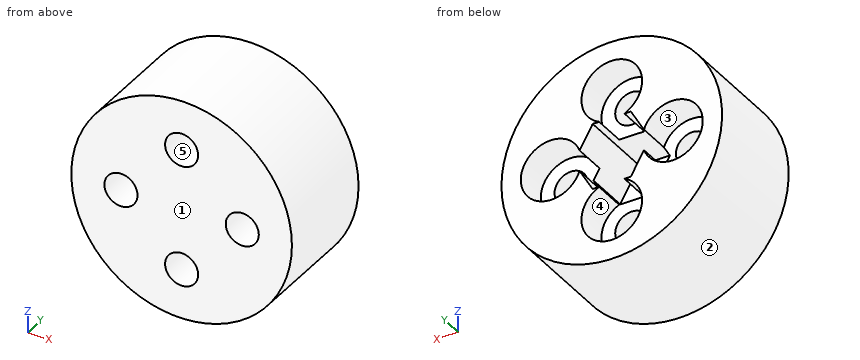
from build123d import *

# Parameters (mm, degrees)
SKETCH1_R           = 10
SKETCH1_R_2         = 1.5
BOSS_EXTRUDE1_DEPTH = 10
SKETCH2_R           = 2.75
CUT_EXTRUDE1_DEPTH  = 3
CUT_EXTRUDE2_DEPTH  = 7


with BuildPart() as part:
    # Sketch1 → Boss-Extrude1 (new body)
    with BuildSketch(Plane(origin=(0, 0, 0), x_dir=(1, 0, 0), z_dir=(0, 1, 0))):
        Circle(SKETCH1_R)
        with Locations((0, 5.5)):
            Circle(SKETCH1_R_2, mode=Mode.SUBTRACT)
        with Locations((5.5, 0)):
            Circle(SKETCH1_R_2, mode=Mode.SUBTRACT)
        with Locations((0, -5.5)):
            Circle(SKETCH1_R_2, mode=Mode.SUBTRACT)
        with Locations((-5.5, 0)):
            Circle(SKETCH1_R_2, mode=Mode.SUBTRACT)
    extrude(amount=BOSS_EXTRUDE1_DEPTH)

    # Sketch2 → Cut-Extrude1 (cut)
    with BuildSketch(Plane(origin=(0, 10, 0), x_dir=(1, 0, 0), z_dir=(0, 1, 0))):
        with Locations((0, 5.5)):
            Circle(SKETCH2_R)
        with Locations((5.5, 0)):
            Circle(SKETCH2_R)
        with Locations((0, -5.5)):
            Circle(SKETCH2_R)
        with Locations((-5.5, 0)):
            Circle(SKETCH2_R)
    extrude(amount=-CUT_EXTRUDE1_DEPTH, mode=Mode.SUBTRACT)

    # Sketch3 → Cut-Extrude2 (cut)
    with BuildSketch(Plane(origin=(0, 10, 0), x_dir=(1, 0, 0), z_dir=(0, 1, 0))):
        Polygon((3.464101615, 0), (1.732050808, 3), (-1.732050808, 3), (-3.464101615, 0), (-1.732050808, -3), (1.732050808, -3), align=None)
    extrude(amount=-CUT_EXTRUDE2_DEPTH, mode=Mode.SUBTRACT)


solid = part.part
The listing builds one solid part. Answer for the finished solid, in the listing's coordinates (mm). Face numbers are marked on the shaded views. A direction names the side the tool comes from. Give positions to 0.01 mm unless a question says otherwise; leave off trailing zeros. Order: outer loops, then holes, each group sorted by start corner. A loop starts at its lowest first (then second) coordinate and runs counter-clockwise, first axis right, second up. Notation, with made-up numbers: (86, -30.75) - (95, -30.75) arc R17 ccw to (95, -0.75) - close; hole circle Ø7 at (82, 37.25). An arc over 180 degrees is marked (long way). Use one line per item in the form item = value.
1) For the marked faces 4 and 5, determine the directions among +Z, -Z, +X, -X, +Y, -Y from which every point of the face is accessible in a straight line to the end or side of a thin tool.
Verdict:
face_4 = +Y
face_5 = +Y, -Y
2) Find section B-B on y = 6.25. Determine the outline of the cut face in (x, z), and give its area (3 significant figures).
Verdict:
outline = circle Ø20 at (0, 0); hole circle Ø3 at (-5.5, 0); hole (-3.46, 0) - (-1.73, -3) - (1.73, -3) - (3.46, 0) - (1.73, 3) - (-1.73, 3) - close; hole circle Ø3 at (0, -5.5); hole circle Ø3 at (0, 5.5); hole circle Ø3 at (5.5, 0)
area = 255 mm^2
3) Consider probe 1 along Z at (x, y) = (0, 3.75); probe 2 along X at (y, z) = (2.5, 0); probe 3 along X at (y, z) = (7.75, -2.5). Determine where each line is inside the solid, lowest interval first. Write a range as [from, to].
Verdict:
probe_1 = [-10, -7], [-4, -3], [3, 4], [7, 10]
probe_2 = [-10, -7], [-4, 4], [7, 10]
probe_3 = [-9.68, -6.65], [-4.35, -2.02], [2.02, 4.35], [6.65, 9.68]
4) Each of these flat-tipped pins is pushed along its axis until it touches: pin 1 (3 mm diameter, centred on x = -1.5, z = -7.5, fed in from +Y); pin 2 (3.5 mm diameter, centred on x = 5.5, z = 0, fed in from +Y); pin 3 (1.8 mm diameter, centred on x = 0, z = 5.5, fed in from +Y); pin 4 (1.5 mm diameter, centred on x = 2, y = 2, fed in from -Z). Where does it stop, or does it pass through?
Verdict:
pin_1 = 10
pin_2 = 7
pin_3 = through
pin_4 = -9.92
5) Find section D-D on z = 5.5. Determine the outline of the cut face in (x, y).
Verdict:
outline = (-8.35, 0) - (-1.5, 0) - (-1.5, 7) - (-2.75, 7) - (-2.75, 10) - (-8.35, 10) - close; (1.5, 0) - (8.35, 0) - (8.35, 10) - (2.75, 10) - (2.75, 7) - (1.5, 7) - close
6) Find section A-A on x = 0. Determine the outline of the cut face in (y, z), and give its area (3 significant figures).
Verdict:
outline = (0, -10) - (10, -10) - (10, -8.25) - (7, -8.25) - (7, -7) - (0, -7) - close; (0, -4) - (7, -4) - (7, -3) - (3, -3) - (3, 3) - (7, 3) - (7, 4) - (0, 4) - close; (0, 7) - (7, 7) - (7, 8.25) - (10, 8.25) - (10, 10) - (0, 10) - close
area = 84.5 mm^2
7) Find section C-C on x = 5.5. Determine the outline of the cut face in (y, z).
Verdict:
outline = (0, -8.35) - (10, -8.35) - (10, -2.75) - (7, -2.75) - (7, -1.5) - (0, -1.5) - close; (0, 1.5) - (7, 1.5) - (7, 2.75) - (10, 2.75) - (10, 8.35) - (0, 8.35) - close
8) The mould has two halves that part along Z. Classify the marked faces 1, 2 and 3: released by +Z, released by -Z, zero draft, split by the parting line, or undercut.
Verdict:
face_1 = zero draft
face_2 = split by the parting line
face_3 = undercut
